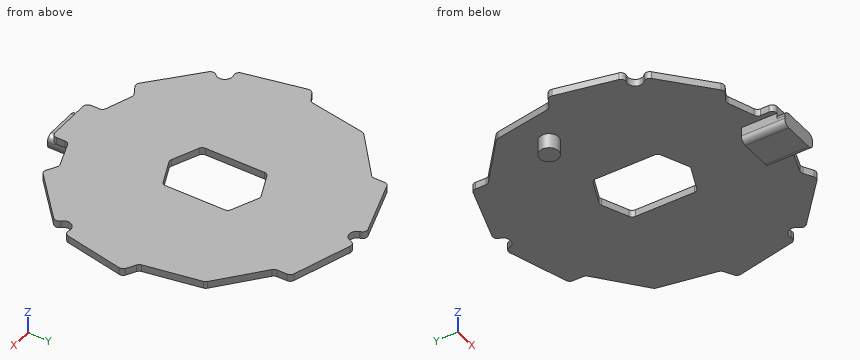
from build123d import *

# Parameters (mm, degrees)
BOSS_EXTRUDE1_DEPTH = 1.5
CUT_EXTRUDE1_DEPTH  = 2.5
CIRPATTERN1_COUNT   = 3
FILLET1_R           = 1
BOSS_EXTRUDE2_DEPTH = 3.17
FILLET2_R           = 1.3
SKETCH5_R           = 2
BOSS_EXTRUDE3_DEPTH = 3.17


with BuildPart() as part:
    # Sketch1 → Boss-Extrude1 (new body)
    with BuildSketch(Plane.XY):
        Polygon((7.362742618, 62.70624455), (-2.408800458, 54.506946358), (-4.623829447, 41.944892725), (-7.530430409, 40.266765877), (-4.165710563, 24.153038268), (8.106826973, 13.1822416), (11.013427935, 14.860368448), (17.5, 12.499449294), (17.5, 9), (28.5, 9), (28.5, 12.499449294), (34.986572065, 14.860368448), (37.893173027, 13.1822416), (50.165710563, 24.153038268), (53.530430409, 40.266765877), (50.623829447, 41.944892725), (48.408800458, 54.506946358), (38.637257382, 62.70624455), (38.637257382, 66.062498246), (23, 71.205429186), (7.362742618, 66.062498246), align=None)
        Polygon((23, 49.472293945), (16.618365096, 46.737307558), (16.618365096, 32.93702959), (23, 30.202043203), (29.381634904, 32.93702959), (29.381634904, 46.737307558), align=None, mode=Mode.SUBTRACT)
    extrude(amount=BOSS_EXTRUDE1_DEPTH)

    # Sketch2 → Cut-Extrude1 (cut, through all)
    with BuildSketch(Plane.XY.offset(1.5)):
        with BuildLine():
            Line((-4.580131881, 26.137712338), (-3.307805549, 26.403387777))
            ThreePointArc((-3.307805549, 26.403387777), (-1.595121467, 25.637168574), (-1.787898214, 23.770831049))
            Line((-1.787898214, 23.770831049), (-2.654143059, 22.801801844))
            Line((-2.654143059, 22.801801844), (-4.165710563, 24.153038268))
            Line((-4.165710563, 24.153038268), (-4.580131881, 26.137712338))
        make_face()
    cut_extrude1 = extrude(amount=-CUT_EXTRUDE1_DEPTH, mode=Mode.SUBTRACT)

    # CirPattern1: Cut-Extrude1 ×3 about axis
    cirpattern1_axis = Axis((23, 39.837168574, 0), (0, 0, 1))
    for i in range(1, CIRPATTERN1_COUNT):
        add(cut_extrude1.rotate(cirpattern1_axis, i * 360 / CIRPATTERN1_COUNT), mode=Mode.SUBTRACT)

    # Fillet1
    fillet1_edges = [part.edges().sort_by_distance(p)[0] for p in [
        (48.654143059, 22.801801844, 0.75),
        (50.580131881, 26.137712338, 0.75),
        (24.925988822, 70.571991541, 0.75),
        (21.074011178, 70.571991541, 0.75),
        (7.362742618, 66.062498246, 0.75),
        (38.637257382, 66.062498246, 0.75),
        (38.637257382, 62.70624455, 0.75),
        (48.408800458, 54.506946358, 0.75),
        (50.623829447, 41.944892725, 0.75),
        (53.530430409, 40.266765877, 0.75),
        (37.893173027, 13.1822416, 0.75),
        (34.986572065, 14.860368448, 0.75),
        (28.5, 12.499449294, 0.75),
        (28.5, 9, 0.75),
        (17.5, 9, 0.75),
        (17.5, 12.499449294, 0.75),
        (11.013427935, 14.860368448, 0.75),
        (8.106826973, 13.1822416, 0.75),
        (-7.530430409, 40.266765877, 0.75),
        (-4.623829447, 41.944892725, 0.75),
        (-2.408800458, 54.506946358, 0.75),
        (7.362742618, 62.70624455, 0.75),
        (16.618365096, 32.93702959, 0.75),
        (23, 30.202043203, 0.75),
        (29.381634904, 32.93702959, 0.75),
        (29.381634904, 46.737307558, 0.75),
        (23, 49.472293945, 0.75),
        (16.618365096, 46.737307558, 0.75),
        (-4.580131881, 26.137712338, 0.75),
        (-2.654143059, 22.801801844, 0.75),
    ]]
    fillet(fillet1_edges, radius=FILLET1_R)

    # Sketch4 → Boss-Extrude2 (add)
    with BuildSketch(Plane(origin=(0, 0, 0), x_dir=(-1, 0, 0), z_dir=(0, 0, -1))):
        Polygon((-27.47, 9), (-27.47, 7.38), (-18.53, 7.38), (-18.53, 9), (-18.53, 16.55), (-27.47, 16.55), align=None)
    extrude(amount=BOSS_EXTRUDE2_DEPTH)

    # Fillet2
    fillet2_edges = [part.edges().sort_by_distance(p)[0] for p in [
        (27.47, 8.19, 0),
        (18.53, 8.19, 0),
        (27.47, 11.965, -3.17),
        (18.53, 11.965, -3.17),
    ]]
    fillet(fillet2_edges, radius=FILLET2_R)

    # Sketch5 → Boss-Extrude3 (add)
    with BuildSketch(Plane(origin=(0, 0, 0), x_dir=(-1, 0, 0), z_dir=(0, 0, -1))):
        with Locations((-2.99, 46.937168574)):
            Circle(SKETCH5_R)
    extrude(amount=BOSS_EXTRUDE3_DEPTH)


solid = part.part
For this review, take the finished solid that the model builds, in its own axes (mm). Round coordinates to 2 decimals unless told otherwise and drop trailing zeros. Order: outer loops, then holes, each group sorted by start corner. A loop starts at its lowest first (then second) coordinate and runs counter-clockwise, first axis right, second up. Notation, with made-up numbers: (51, 64) -> (76, 64) arc R18 ccw to (76, 77) -> close; hole circle Ø3 at (51.25, -32.75). An arc over 180 degrees is marked (long way). Put each result on its own line as item: value.
Q1. Add section C-C on x = 13. Write out the cut boundary in (y, z), plus the area to 3 significant figures.
Check result:
outline: (14.14, 0) -> (67.92, 0) -> (67.92, 1.5) -> (14.14, 1.5) -> close
area: 80.7 mm2
Q2. For probe 1 along Z at (x, y) = (9, 17.5); probe 2 along X at (y, z) = (65.5, 0.45); probe 3 along X at (y, z) = (36, 0.5), list the stretches that pass through material, from the lowest coordinate up. Write a range as [from, to].
Check result:
probe 1: [0, 1.5]
probe 2: [7.38, 38.62]
probe 3: [-6.64, 16.62], [29.38, 52.64]
Q3. Insertion check: pin 1 Ø1.6 at (y, z) = (65, 0.5) entering from +X; pin 2 Ø0.8 at (y, z) = (37, 1) entering from -X; pin 3 Ø1.2 at (y, z) = (64, 1) entering from -X; pin 4 Ø1 at (x, z) = (46.5, -1) entering from +Y. Each pin has a flat end and moves straight along its axis. Give the tip position at first contact, or say it passes through.
Check result:
pin 1: x = 38.64
pin 2: x = -6.93
pin 3: x = 7.36
pin 4: through
Q4. Add section B-B on x = 2.99. Write out the cut boundary in (y, z).
Check result:
outline: (17.76, 0) -> (44.94, 0) -> (44.94, -3.17) -> (48.94, -3.17) -> (48.94, 0) -> (59.04, 0) -> (59.04, 1.5) -> (17.76, 1.5) -> close
Q5. Add section A-A on y = 36.5. Write out the cut boundary in (x, z).
Check result:
outline: (-6.74, 0) -> (16.62, 0) -> (16.62, 1.5) -> (-6.74, 1.5) -> close; (29.38, 0) -> (52.74, 0) -> (52.74, 1.5) -> (29.38, 1.5) -> close
